Design review of the part built by this model. Coordinates are the model's own, in mm. Face numbers are marked on the shaded views. Give positions to 0.01 mm unless a question says otherwise; leave off trailing zeros. Write each loop counter-clockwise with the first axis right and the second up, starting at its lowest first coordinate (ties: lowest second). Pieces come first, ordered by that corner, then holes. Notation, with made-up numbers: M 9,-31.75 L 52,-31.75 A16 cw 52,-11.75 Z; hole C 28,-14.75 d2. An arc over 180 degrees is marked long. Answer in a Markdown table with one row per item.
Autodesk Inventor part; units mm, degrees
ref_plane "YZ Plane" through (0, 0, 0) normal (1, 0, 0) x (0, 1, 0)
ref_plane "XZ Plane" through (0, 0, 0) normal (0, 1, 0) x (-1, 0, 0)
ref_plane "XY Plane" through (0, 0, 0) normal (0, 0, 1) x (1, 0, 0)
sketch "Sketch1" plane through (0, 0, 0) normal (0, 0, 1) x (1, 0, 0)
  circle A0 centre (0, 0) radius 10
  line L0 (0, 0) -> (-46, 0) construction
  circle A1 centre (-46, 0) radius 10
  line L1 (-46, 10) -> (0, 10)
  line L2 (-46, -10) -> (0, -10)
  dimension "d0" = 20
  dimension "d1" = 20
  dimension "d2" = 46
extrude "Extrusion1" add sketch "Sketch1" along normal mid plane 3.5
hole "Hole3" at (-46, 0, 1.75) direction (0, 0, -1) diameter 8 end through all
hole "Hole4" at (0, 0, 1.75) direction (0, 0, -1) diameter 9 end through all
properties part number "201-12" material "Steel"
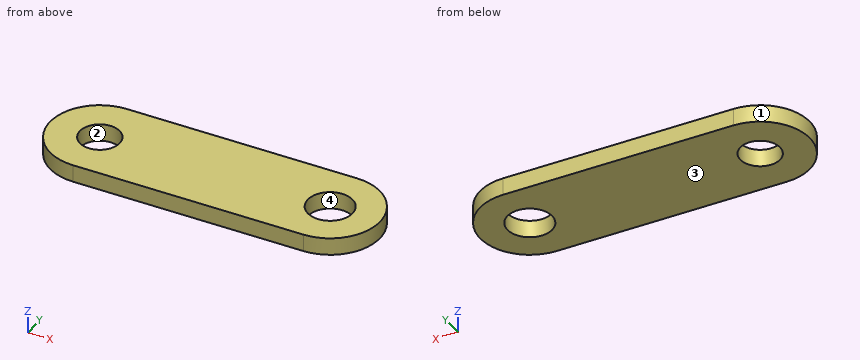
1) Add section B-B (x = -3.5). Write out the cut boundary in (y, z), and give its area (3 significant figures).
Geometry says:
| item | result |
|---|---|
| outline | M -10,-1.75 L -2.83,-1.75 L -2.83,1.75 L -10,1.75 Z; M 2.83,-1.75 L 10,-1.75 L 10,1.75 L 2.83,1.75 Z |
| area | 50.2 mm^2 |
2) Add section D-D (y = -7.75). Write out the cut boundary in (x, z).
Geometry says:
| item | result |
|---|---|
| outline | M -52.32,-1.75 L 6.32,-1.75 L 6.32,1.75 L -52.32,1.75 Z |
3) The part is to be moulded in two halves that separate along X. For the marked faces 1, 2, 3 and 4, say which applies: released by +X, released by -X, zero draft, split by the parting line, or undercut.
Geometry says:
| item | result |
|---|---|
| face 1 | released by -X |
| face 2 | undercut |
| face 3 | zero draft |
| face 4 | undercut |
4) To check wall thickness, follow probe 1 along X at (y, z) = (0, 0.75); probe 2 along X at (y, z) = (1.25, 1.15); probe 3 along Y at (x, z) = (0, 0.7). State the ranges of each line that lie inside material, in increasing order. Write a range as [from, to].
Geometry says:
| item | result |
|---|---|
| probe 1 | [-56, -50], [-42, -4.5], [4.5, 10] |
| probe 2 | [-55.92, -49.8], [-42.2, -4.32], [4.32, 9.92] |
| probe 3 | [-10, -4.5], [4.5, 10] |
5) Add section A-A (y = 0). Write out the cut boundary in (x, z).
Geometry says:
| item | result |
|---|---|
| outline | M -56,-1.75 L -50,-1.75 L -50,1.75 L -56,1.75 Z; M -42,-1.75 L -4.5,-1.75 L -4.5,1.75 L -42,1.75 Z; M 4.5,-1.75 L 10,-1.75 L 10,1.75 L 4.5,1.75 Z |
6) Add section C-C (z = 0.2). Write out the cut boundary in (x, y).
Geometry says:
| item | result |
|---|---|
| outline | M -46,-10 L 0,-10 A10 ccw 0,10 L -46,10 A10 ccw Z; hole C -46,0 d8; hole C 0,0 d9 |
7) Insertion check: P1, Ø1, axis at x = 2, z = -1, coming from the -Y side; P2, Ø1, axis at y = -3.5, z = -1, coming from the +X side. Each pin has a flat end and moves straight along its axis. Give the tip position at first contact, or say it passes through.
Geometry says:
| item | result |
|---|---|
| P1 | y = -9.89 |
| P2 | x = 9.54 |
